Work out the finished part from the listing and answer in its coordinate system (mm). Face numbers are marked on the shaded views. Round coordinates to 2 decimals unless told otherwise and drop trailing zeros. Order: outer loops, then holes, each group sorted by start corner. A loop starts at its lowest first (then second) coordinate and runs counter-clockwise, first axis right, second up. Notation, with made-up numbers: (43, -7) - (82, -7) arc R10 cw to (82, 2) - close; hole circle Ø5 at (41, 12.5). An arc over 180 degrees is marked (long way). Use CSV: the item, a comma, the result in double quotes.
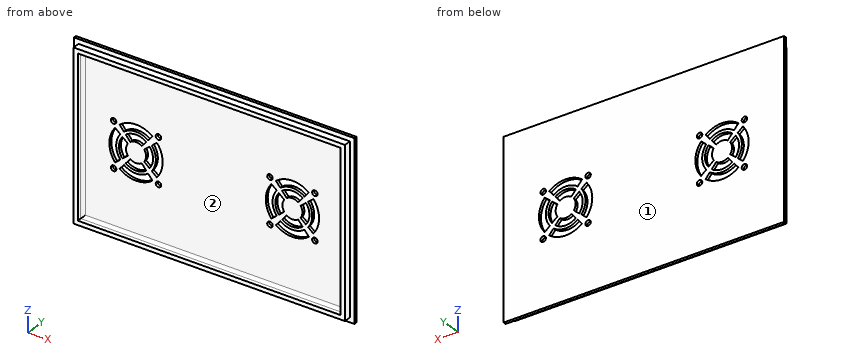
from build123d import *

# Parameters (mm, degrees)
SKETCH1_W              = 200
SKETCH1_H              = 125.5
BOSS_EXTRUDE1_DEPTH    = 2
SKETCH2_W              = 193.5
SKETCH2_H              = 119
BOSS_EXTRUDE2_DEPTH    = 5
SKETCH3_W              = 187.5
SKETCH3_H              = 113
CUT_EXTRUDE1_DEPTH     = 5
FILLET1_R              = 2
M3_5_CLEARANCE_HOLE1_D = 3.9
CUT_EXTRUDE3_DEPTH     = 2
LPATTERN1_COUNT        = 2
LPATTERN1_PITCH        = 111.5


with BuildPart() as part:
    # Sketch1 → Boss-Extrude1 (new body)
    with BuildSketch(Plane(origin=(0, 0, 0), x_dir=(1, 0, 0), z_dir=(0, 1, 0))):
        with Locations((11.680911681, -22.009259259)):
            Rectangle(SKETCH1_W, SKETCH1_H)
    extrude(amount=BOSS_EXTRUDE1_DEPTH)

    # Sketch2 → Boss-Extrude2 (add)
    with BuildSketch(Plane.XZ):
        with Locations((11.680911681, 22.009259259)):
            Rectangle(SKETCH2_W, SKETCH2_H)
    extrude(amount=BOSS_EXTRUDE2_DEPTH)

    # Sketch3 → Cut-Extrude1 (cut)
    with BuildSketch(Plane.XZ.offset(5)):
        with Locations((11.680911681, 22.009259259)):
            Rectangle(SKETCH3_W, SKETCH3_H)
    extrude(amount=-CUT_EXTRUDE1_DEPTH, mode=Mode.SUBTRACT)

    # Fillet1
    fillet1_edges = [part.edges().sort_by_distance(p)[0] for p in [
        (105.430911681, 0, 22.009259259),
        (11.680911681, 0, -34.490740741),
        (-82.069088319, 0, 22.009259259),
        (11.680911681, 0, 78.509259259),
    ]]
    fillet(fillet1_edges, radius=FILLET1_R)

    # M3.5 Clearance Hole1 (through all)
    with Locations(Plane(origin=(0, 2, 0), x_dir=(-1, 0, 0), z_dir=(0, 1, 0))):
        with Locations((60.069088319, 38.009259259), (28.069088319, 38.009259259), (28.069088319, 6.009259259), (60.069088319, 6.009259259), (-51.430911681, 38.009259259), (-51.430911681, 6.009259259), (-83.430911681, 6.009259259), (-83.430911681, 38.009259259)):
            Hole(M3_5_CLEARANCE_HOLE1_D / 2)

    # Sketch9 → Cut-Extrude3 (cut)
    with BuildSketch(Plane(origin=(0, 2, 0), x_dir=(1, 0, 0), z_dir=(0, 1, 0))):
        with BuildLine():
            Line((-59.006386494, -10.267150282), (-55.293048336, -13.388835035))
            ThreePointArc((-55.293048336, -13.388835035), (-58.221436969, -22.013724686), (-55.287606174, -30.636764657))
            Line((-55.287606174, -30.636764657), (-59.006386494, -33.751368237))
            ThreePointArc((-59.006386494, -33.751368237), (-63.069088319, -22.009259259), (-59.006386494, -10.267150282))
        make_face()
        with BuildLine():
            Line((-53.75963561, -14.677926123), (-49.910160311, -17.914057022))
            ThreePointArc((-49.910160311, -17.914057022), (-51.202718747, -22.020227048), (-49.897540172, -26.122403114))
            Line((-49.897540172, -26.122403114), (-53.752014553, -29.350655033))
            ThreePointArc((-53.752014553, -29.350655033), (-56.220430324, -22.015570701), (-53.75963561, -14.677926123))
        make_face()
        with BuildLine():
            Line((-52.696593717, -10.790741404), (-55.811197297, -7.071961085))
            ThreePointArc((-55.811197297, -7.071961085), (-44.069088319, -3.009259259), (-32.326979341, -7.071961085))
            Line((-32.326979341, -7.071961085), (-35.448664095, -10.785299243))
            ThreePointArc((-35.448664095, -10.785299243), (-44.073553746, -7.856910609), (-52.696593717, -10.790741404))
        make_face()
        with BuildLine():
            Line((-48.182232174, -16.180807406), (-51.410484093, -12.326333025))
            ThreePointArc((-51.410484093, -12.326333025), (-44.075399761, -9.857917254), (-36.737755183, -12.318711968))
            Line((-36.737755183, -12.318711968), (-39.973886082, -16.168187268))
            ThreePointArc((-39.973886082, -16.168187268), (-44.080056108, -14.875628831), (-48.182232174, -16.180807406))
        make_face()
        with BuildLine():
            Line((-32.850570464, -13.381753861), (-29.131790144, -10.267150282))
            ThreePointArc((-29.131790144, -10.267150282), (-25.069088319, -22.009259259), (-29.131790144, -33.751368237))
            Line((-29.131790144, -33.751368237), (-32.845128303, -30.629683483))
            ThreePointArc((-32.845128303, -30.629683483), (-29.916739669, -22.004793832), (-32.850570464, -13.381753861))
        make_face()
        with BuildLine():
            Line((-38.240636466, -17.896115404), (-34.386162085, -14.667863485))
            ThreePointArc((-34.386162085, -14.667863485), (-31.917746314, -22.002947817), (-34.378541028, -29.340592396))
            Line((-34.378541028, -29.340592396), (-38.228016328, -26.104461496))
            ThreePointArc((-38.228016328, -26.104461496), (-36.935457891, -21.998291471), (-38.240636466, -17.896115404))
        make_face()
        with BuildLine():
            Line((-35.441582921, -33.227777114), (-32.326979341, -36.946557434))
            ThreePointArc((-32.326979341, -36.946557434), (-44.069088319, -41.009259259), (-55.811197297, -36.946557434))
            Line((-55.811197297, -36.946557434), (-52.689512543, -33.233219276))
            ThreePointArc((-52.689512543, -33.233219276), (-44.064622892, -36.161607909), (-35.441582921, -33.227777114))
        make_face()
        with BuildLine():
            Line((-39.955944464, -27.837711112), (-36.727692545, -31.692185493))
            ThreePointArc((-36.727692545, -31.692185493), (-44.062776877, -34.160601264), (-51.400421455, -31.69980655))
            Line((-51.400421455, -31.69980655), (-48.164290556, -27.850331251))
            ThreePointArc((-48.164290556, -27.850331251), (-44.058120531, -29.142889687), (-39.955944464, -27.837711112))
        make_face()
    cut_extrude3 = extrude(amount=-CUT_EXTRUDE3_DEPTH, mode=Mode.SUBTRACT)

    # LPattern1: Cut-Extrude3 ×2
    with Locations(*[(i * LPATTERN1_PITCH, 0, 0) for i in range(1, LPATTERN1_COUNT)]):
        add(cut_extrude3, mode=Mode.SUBTRACT)


solid = part.part
(1) Each of these flat-tipped pins is pushed along its axis until it touches: pin 1 (2.5 mm diameter, centred on y = -2.5, z = 15.5, fed in from +X); pin 2 (3.5 mm diameter, centred on y = -3, z = 49.5, fed in from -X); pin 3 (1.5 mm diameter, centred on x = 9, y = -3, fed in from -Z); pin 4 (5 mm diameter, centred on x = 51.43, z = 38.01, fed in from +Y). Where does it stop, or does it pass through?
Findings below:
pin 1,"stops at x = 108.43"
pin 2,"stops at x = -85.07"
pin 3,"stops at z = -37.49"
pin 4,"stops at y = 2"
(2) The mould has two halves that part along X. Classify the marked faces 1 and 2: released by +X, released by -X, zero draft, split by the parting line, or undercut.
Findings below:
face 1,"zero draft"
face 2,"undercut"
(3) Find section D-D (z = 50.5). Determine the outline of the cut face in (x, y), and give its area (3 significant figures).
Findings below:
outline,"(-88.32, 0) - (-85.07, 0) - (-85.07, -5) - (-82.07, -5) - (-82.07, -2) arc R2 cw to (-80.07, 0) - (103.43, 0) arc R2 cw to (105.43, -2) - (105.43, -5) - (108.43, -5) - (108.43, 0) - (111.68, 0) - (111.68, 2) - (-88.32, 2) - close"
area,"432 mm²"
(4) Find section A-A (y = -3.75). Determine the outline of the cut face in (x, z).
Findings below:
outline,"(-85.07, -37.49) - (108.43, -37.49) - (108.43, 81.51) - (-85.07, 81.51) - close; hole (-82.07, -34.49) - (105.43, -34.49) - (105.43, 78.51) - (-82.07, 78.51) - close"
(5) Find section C-C (x = 33.5). Determine the outline of the cut face in (y, z).
Findings below:
outline,"(-5, -37.49) - (0, -37.49) - (0, -40.74) - (2, -40.74) - (2, 84.76) - (0, 84.76) - (0, 81.51) - (-5, 81.51) - (-5, 78.51) - (-2, 78.51) arc R2 cw to (0, 76.51) - (0, -32.49) arc R2 cw to (-2, -34.49) - (-5, -34.49) - close"
(6) Find the intervals of material crossed by L1, parallel to X at y = -2.5, z = 1; L2, parallel to Z at x = 10.5, y = -1.75; L3, parallel to Y at x = 16.5, z = 35, in increasing order. Write a range as from..to.
Findings below:
L1,"x = -85.07..-82.07, 105.43..108.43"
L2,"z = -37.49..-34.48, 78.49..81.51"
L3,"y = 0..2"
(7) Find section B-B (x = -42). State how many separate pieces and enclosed holes the cut face has, and give its area (3 significant figures).
Findings below:
separate pieces,"5"
enclosed holes,"0"
area,"243 mm²"
